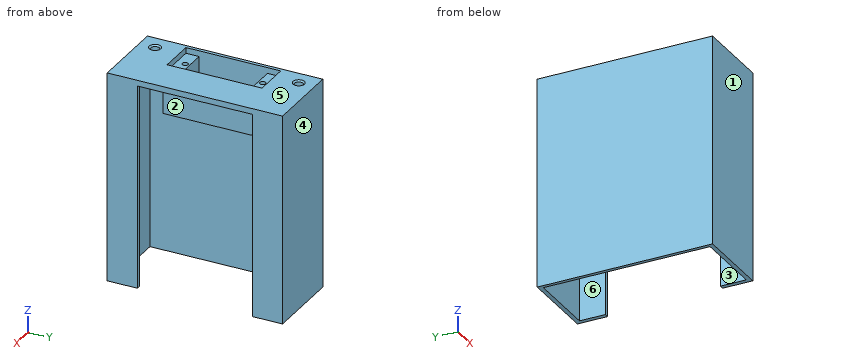
```python
from build123d import *

# Parameters (mm, degrees)
SKETCH_1_W           = 73
SKETCH_1_H           = 61
EXTRUDE_1_DEPTH      = 1.5
SKETCH_3_W           = 73
SKETCH_3_H           = 1.5
EXTRUDE_2_DEPTH      = 24
SKETCH_4_W           = 24
SKETCH_4_H           = 58
EXTRUDE_8_DEPTH      = 2
SKETCH_18_W          = 12
SKETCH_18_H          = 23
CUT_EXTRUDE_10_DEPTH = 2
SKETCH_19_W          = 12
SKETCH_19_H          = 6
EXTRUDE_9_DEPTH      = 15
SKETCH_21_W          = 1
SKETCH_21_H          = 35
EXTRUDE_10_DEPTH     = 15
SKETCH_24_W          = 12
SKETCH_24_H          = 5
CUT_EXTRUDE_12_DEPTH = 2
SKETCH_25_R          = 1
CUT_EXTRUDE_13_DEPTH = 10
SKETCH_28_W          = 73
SKETCH_28_H          = 10.5
EXTRUDE_11_DEPTH     = 1.5
SKETCH_31_W          = 2
SKETCH_31_H          = 40
EXTRUDE_12_DEPTH     = 1.5
SKETCH_32_R          = 1.5
CUT_EXTRUDE_14_DEPTH = 5
CHAMFER_1_SIZE       = 0.5
CHAMFER_2_SIZE       = 0.5
SKETCH_33_W          = 12
SKETCH_33_H          = 23
CUT_EXTRUDE_15_DEPTH = 48
SKETCH_34_W          = 0.3
SKETCH_34_H          = 58
CUT_EXTRUDE_16_DEPTH = 56
SKETCH_35_W          = 0.3
SKETCH_35_H          = 11.5
CUT_EXTRUDE_17_DEPTH = 15
SKETCH_36_W          = 12.6
SKETCH_36_H          = 4.6
CUT_EXTRUDE_18_DEPTH = 2


with BuildPart() as part:
    # 草图1 → 凸台-拉伸1 (new body)
    with BuildSketch(Plane(origin=(0, 0, 0), x_dir=(0, 0, -1), z_dir=(1, 0, 0))):
        Rectangle(SKETCH_1_W, SKETCH_1_H)
    extrude(amount=-EXTRUDE_1_DEPTH)

    # 草图3 → 凸台-拉伸2 (add)
    with BuildSketch(Plane(origin=(0, 0, 0), x_dir=(0, 0, -1), z_dir=(1, 0, 0))):
        with Locations((0, 29.75)):
            Rectangle(SKETCH_3_W, SKETCH_3_H)
        with Locations((0, -29.75)):
            Rectangle(SKETCH_3_W, SKETCH_3_H)
    extrude(amount=EXTRUDE_2_DEPTH)

    # 草图4 → 凸台-拉伸8 (add)
    with BuildSketch(Plane.XY.offset(36.5)):
        with Locations((12, 0)):
            Rectangle(SKETCH_4_W, SKETCH_4_H)
    extrude(amount=-EXTRUDE_8_DEPTH)

    # 草图18 → 切除-拉伸10 (cut)
    with BuildSketch(Plane(origin=(0, 0, 34.5), x_dir=(-1, 0, 0), z_dir=(0, 0, -1))):
        with Locations((-6, 0)):
            Rectangle(SKETCH_18_W, SKETCH_18_H)
    extrude(amount=-CUT_EXTRUDE_10_DEPTH, mode=Mode.SUBTRACT)

    # 草图19 → 凸台-拉伸9 (add)
    with BuildSketch(Plane(origin=(0, 0, 34.5), x_dir=(-1, 0, 0), z_dir=(0, 0, -1))):
        with Locations((-6, 14.5)):
            Rectangle(SKETCH_19_W, SKETCH_19_H)
        with Locations((-6, -14.5)):
            Rectangle(SKETCH_19_W, SKETCH_19_H)
    extrude(amount=EXTRUDE_9_DEPTH)

    # 草图21 → 凸台-拉伸10 (add)
    with BuildSketch(Plane(origin=(0, 0, 34.5), x_dir=(-1, 0, 0), z_dir=(0, 0, -1))):
        with Locations((-12.5, 0)):
            Rectangle(SKETCH_21_W, SKETCH_21_H)
    extrude(amount=EXTRUDE_10_DEPTH)

    # 草图24 → 切除-拉伸12 (cut)
    with BuildSketch(Plane.XY.offset(36.5)):
        with Locations((6, 14)):
            Rectangle(SKETCH_24_W, SKETCH_24_H)
        with Locations((6, -14)):
            Rectangle(SKETCH_24_W, SKETCH_24_H)
    extrude(amount=-CUT_EXTRUDE_12_DEPTH, mode=Mode.SUBTRACT)

    # 草图25 → 切除-拉伸13 (cut)
    with BuildSketch(Plane.XY.offset(34.5)):
        with Locations((6, 13.5)):
            Circle(SKETCH_25_R)
        with Locations((6, -13.5)):
            Circle(SKETCH_25_R)
    extrude(amount=-CUT_EXTRUDE_13_DEPTH, mode=Mode.SUBTRACT)

    # 草图28 → 凸台-拉伸11 (add)
    with BuildSketch(Plane(origin=(24, 0, 0), x_dir=(0, 0, -1), z_dir=(1, 0, 0))):
        with Locations((0, 25.25)):
            Rectangle(SKETCH_28_W, SKETCH_28_H)
        with Locations((0, -25.25)):
            Rectangle(SKETCH_28_W, SKETCH_28_H)
    extrude(amount=EXTRUDE_11_DEPTH)

    # 草图31 → 凸台-拉伸12 (add)
    with BuildSketch(Plane(origin=(24, 0, 0), x_dir=(0, 0, -1), z_dir=(1, 0, 0))):
        with Locations((-35.5, 0)):
            Rectangle(SKETCH_31_W, SKETCH_31_H)
    extrude(amount=EXTRUDE_12_DEPTH)

    # 草图32 → 切除-拉伸14 (cut)
    with BuildSketch(Plane(origin=(0, 0, 34.5), x_dir=(-1, 0, 0), z_dir=(0, 0, -1))):
        with Locations((-4, 25)):
            Circle(SKETCH_32_R)
        with Locations((-4, -25)):
            Circle(SKETCH_32_R)
    extrude(amount=-CUT_EXTRUDE_14_DEPTH, mode=Mode.SUBTRACT)

    # 倒角1
    chamfer_1_edges = [part.edges().sort_by_distance(p)[0] for p in [
        (5.5, 25, 36.5),
    ]]
    chamfer(chamfer_1_edges, length=CHAMFER_1_SIZE)

    # 倒角2
    chamfer_2_edges = [part.edges().sort_by_distance(p)[0] for p in [
        (5.5, -25, 36.5),
    ]]
    chamfer(chamfer_2_edges, length=CHAMFER_2_SIZE)

    # 草图33 → 切除-拉伸15 (cut)
    with BuildSketch(Plane(origin=(0, 0, 19.5), x_dir=(-1, 0, 0), z_dir=(0, 0, -1))):
        Polygon((0, 11.9), (-12.3, 11.9), (-12.3, -11.9), (0, -11.9), (0.3, -11.9), (0.3, 11.9), align=None)
        with Locations((-6, 0)):
            Rectangle(SKETCH_33_W, SKETCH_33_H, mode=Mode.SUBTRACT)
    extrude(amount=-CUT_EXTRUDE_15_DEPTH, mode=Mode.SUBTRACT)

    # 草图34 → 切除-拉伸16 (cut)
    with BuildSketch(Plane(origin=(0, 0, -36.5), x_dir=(-1, 0, 0), z_dir=(0, 0, -1))):
        with Locations((0.15, 0)):
            Rectangle(SKETCH_34_W, SKETCH_34_H)
    extrude(amount=-CUT_EXTRUDE_16_DEPTH, mode=Mode.SUBTRACT)

    # 草图35 → 切除-拉伸17 (cut)
    with BuildSketch(Plane(origin=(0, 0, 19.5), x_dir=(-1, 0, 0), z_dir=(0, 0, -1))):
        with Locations((0.15, 23.25)):
            Rectangle(SKETCH_35_W, SKETCH_35_H)
        with Locations((0.15, -23.25)):
            Rectangle(SKETCH_35_W, SKETCH_35_H)
    extrude(amount=-CUT_EXTRUDE_17_DEPTH, mode=Mode.SUBTRACT)

    # 草图36 → 切除-拉伸18 (cut)
    with BuildSketch(Plane.XY.offset(36.5)):
        with Locations((6, -14.2)):
            Rectangle(SKETCH_36_W, SKETCH_36_H)
        with Locations((6, 14.2)):
            Rectangle(SKETCH_36_W, SKETCH_36_H)
    extrude(amount=-CUT_EXTRUDE_18_DEPTH, mode=Mode.SUBTRACT)


solid = part.part
```
Part model, mm, in its own coordinate system. Face numbers are marked on the shaded views. A direction names the side the tool comes from. Round coordinates to 2 decimals unless told otherwise and drop trailing zeros. Order: outer loops, then holes, each group sorted by start corner. A loop starts at its lowest first (then second) coordinate and runs counter-clockwise, first axis right, second up. Notation, with made-up numbers: M 26,15 L 53,15 A30 cw 53,54 Z; hole C -23.5,43.25 d7. An arc over 180 degrees is marked long. Answer in a Markdown table with one row per item. Add a question column.
Q1. 3-axis set-ups, long thin cutter, end or side, ignore diameter. For the marked faces 1, 2 and 3: which of +Z, -Z, +X, -X, +Y, -Y reach the whole face in a straight line?
Q2. Cut at A-A on y = -6. Give the cut face in (x, z), and give its area (4 significant figures).
Q3. Pin check, flat tips, straight feed: pin 1 (1.4 mm diameter, centred on x = 5.5, y = -14, fed in from +Z); pin 2 (8 mm diameter, centred on x = 11, y = -5.5, fed in from -Z); pin 3 (4.5 mm diameter, centred on y = 8.5, z = 24.5, fed in from +X). Stop position of each tip, or through.
Q4. Mould opens along Y. For the marked faces 4, 5 and 6 say: +Y half, -Y half, draft (parallel to the pull), parting line (faces both ways), or undercut.
Q5. Cut at C-C on x = 11.5. Give the cut face in (y, z), and give its area (3 significant figures).
Q6. Cut at B-B on x = 4. Give the number of separate pieces and of enclosed holes in the cut face, and give its area (4 significant figures).
Q7. Cut at D-D on z = 25.5. Give the cut face in (x, y), and give its area (3 significant figures).
Q8. Wall check: L1, parallel to Y at x = 4, z = 35.7; L2, parallel to Y at x = 6, z = 28.5; L3, parallel to Y at x = 5.25, z = 8. Give the ranges that are in metal, low to high. Write a range as from..to.
Established:
| question | item | result |
|---|---|---|
| 1 | face 1 | +Z, -Z, +X, -X, -Y |
| 1 | face 2 | -Z, +X |
| 1 | face 3 | -Z |
| 2 | outline | M -1.5,-36.5 L -0.3,-36.5 L -0.3,36.5 L -1.5,36.5 Z; M 12.3,19.5 L 13,19.5 L 13,34.5 L 25.5,34.5 L 25.5,36.5 L 12.3,36.5 Z |
| 2 | area | 124.5 mm2 |
| 3 | pin 1 | stops at z = 34.5 |
| 3 | pin 2 | stops at z = 19.5 |
| 3 | pin 3 | stops at x = 13 |
| 4 | face 4 | +Y half |
| 4 | face 5 | draft |
| 4 | face 6 | undercut |
| 5 | outline | M -30.5,-36.5 L -29,-36.5 L -29,34.5 L -17.5,34.5 L -17.5,19.5 L -11.9,19.5 L -11.9,34.5 L -16.5,34.5 L -16.5,36.5 L -30.5,36.5 Z; M 11.9,19.5 L 17.5,19.5 L 17.5,34.5 L 29,34.5 L 29,-36.5 L 30.5,-36.5 L 30.5,36.5 L 16.5,36.5 L 16.5,34.5 L 11.9,34.5 Z |
| 5 | area | 437 mm2 |
| 6 | separate pieces | 4 |
| 6 | enclosed holes | 0 |
| 6 | area | 424.5 mm2 |
| 7 | outline | M -1.5,-30.5 L 25.5,-30.5 L 25.5,-20 L 24,-20 L 24,-29 L -0.3,-29 L -0.3,-17.5 L 13,-17.5 L 13,17.5 L -0.3,17.5 L -0.3,29 L 24,29 L 24,20 L 25.5,20 L 25.5,30.5 L -1.5,30.5 Z; hole M -0.3,-11.9 L 12.3,-11.9 L 12.3,11.9 L -0.3,11.9 Z; hole C 6,-13.5 d2; hole C 6,13.5 d2 |
| 7 | area | 337 mm2 |
| 8 | L1 | y = -30.5..-26.5, -23.5..-16.5, 16.5..23.5, 26.5..30.5 |
| 8 | L2 | y = -30.5..-29, -17.5..-14.5, -12.5..-11.9, 11.9..12.5, 14.5..17.5, 29..30.5 |
| 8 | L3 | y = -30.5..-29, 29..30.5 |
